from build123d import *

# Parameters (mm, degrees)
F0_W     = 149.987
F0_H     = 69.6976
F1_DEPTH = 25.4
F2_W     = 66.675
F2_H     = 25.2984
F3_DEPTH = 12.7
F5_DEPTH = 12.7
F6_W     = 37.735215
F6_H     = 10.168377
F7_DEPTH = 12.7
F9_DEPTH = 1.3716


with BuildPart() as f1:
    # F0 (on Front) → F1 (new body)
    with BuildSketch(Plane.XZ):
        Rectangle(F0_W, F0_H)
    extrude(amount=F1_DEPTH)

    # F2 (on face) → F3 (cut)
    with BuildSketch(Plane.XZ.offset(25.4)):
        with Locations((0, 22.1996)):
            Rectangle(F2_W, F2_H)
    extrude(amount=-F3_DEPTH, mode=Mode.SUBTRACT)

    # F4 (on face) → F5 (cut)
    with BuildSketch(Plane.XZ.offset(25.4)):
        Polygon((33.3375, 9.5504), (-33.3375, 9.5504), (-74.9935, 15.9512), (-74.9935, -24.998723), (74.9935, -24.998723), (74.9935, 15.9512), align=None)
    extrude(amount=-F5_DEPTH, mode=Mode.SUBTRACT)

    # F6 (on face) → F7 (join)
    with BuildSketch(Plane.XZ.offset(12.7)):
        with Locations((-14.469893, 14.634588)):
            Rectangle(F6_W, F6_H)
    extrude(amount=F7_DEPTH)

    # F8 (on face) → F9 (join)
    with BuildSketch(Plane(origin=(0, 0, 0), x_dir=(-1, 0, 0), z_dir=(0, 1, 0))):
        Polygon((-5.378736, 13.970545), (-13.324757, 27.590852), (-14.065389, 25.489114), (-10.146485, 18.771706), (-11.020009, 17.885251), (-14.361666, 23.663847), (-14.942966, 21.517376), (-11.619632, 15.689826), (-12.511065, 14.787045), (-15.413008, 19.761277), (-16.012603, 17.598834), (-13.045956, 12.513692), (-13.982809, 11.584633), (-16.470851, 15.849397), (-17.257973, 13.296365), (-14.628438, 8.777128), (-15.523009, 7.89), (-17.603708, 11.507705), (-19.224059, 5.78715), (-2.314166, -5.613022), (-2.314166, -7.630318), (-7.419162, -13.35848), (-6.456276, -14.415695), (-3.713523, -11.190438), (-3.327152, -11.61466), (-5.894728, -14.962248), (-4.883376, -15.92657), (-2.861757, -13.310585), (-2.387249, -13.763027), (-4.326059, -16.532207), (-3.442212, -17.475365), (-1.889574, -15.639646), (-1.311372, -16.128685), (-2.922849, -18.03397), (-1.92949, -18.981067), (-1.01934, -17.795069), (-0.374972, -18.382913), (-1.436909, -19.49672), (0.299996, -21.152735), (1.878888, -19.49672), (0.919775, -18.382913), (1.456053, -17.795069), (2.404852, -18.981067), (3.415506, -18.03397), (1.820631, -16.128685), (2.404852, -15.639646), (3.941494, -17.475365), (4.840794, -16.532207), (2.89907, -13.763027), (3.395835, -13.310585), (5.390918, -15.92657), (6.449709, -14.962248), (3.797929, -11.61466), (4.333463, -11.190438), (6.88834, -14.415695), (8.049124, -13.35848), (2.832049, -7.630318), (2.832049, -5.613022), (19.73976, 5.78715), (18.108712, 11.507705), (15.947106, 7.89), (15.048685, 8.777128), (17.748964, 13.296365), (16.968758, 15.849397), (14.510422, 11.584633), (13.569537, 12.513692), (16.607948, 17.598834), (15.947106, 19.761277), (12.974964, 14.787045), (12.060693, 15.689826), (15.542698, 21.517376), (14.857555, 23.663847), (11.526601, 17.885251), (10.627024, 18.771706), (14.432989, 25.489114), (13.762125, 27.590852), (5.914255, 13.976232), (9.222287, 8.290899), (5.935366, 5.0631), (2.720125, 5.0631), (4.767341, 7.097367), (2.442414, 11.553886), (-3.681165, 9.865881), (-0.970141, 7.097367), (-3.078866, 5.03243), (-5.430478, 5.03243), (-8.664062, 8.293143), align=None)
        Polygon((-0.485612, 0.682145), (0, 2.126915), (0.485041, 0.682145), (2.099235, 0.682145), (0.796223, -0.344701), (1.207654, -1.78771), (0, -0.84399), (-1.242889, -1.792924), (-0.851036, -0.344701), (-2.131865, 0.682145), align=None, mode=Mode.SUBTRACT)
    extrude(amount=F9_DEPTH)


solid = f1.part
Geometry check sheet. Reference: the model listing, model coordinates, mm. A direction names the side the tool comes from. Coordinates: 2 decimals unless noted, no trailing zeros. Order: outer loops, then holes, each group sorted by start corner. A loop starts at its lowest first (then second) coordinate and runs counter-clockwise, first axis right, second up. Notation, with made-up numbers: (-6.5, -3.5) - (44.5, -3.5) arc R24 ccw to (44.5, 35.5) - close; hole circle Ø1 at (68.5, 17). An arc over 180 degrees is marked (long way). Answer in a Markdown table with one row per item. Add a question column.
1) Cross-section at D-D, the plane x = -60.5. Record the cut outline in (y, z), then the cut area to 3 significant figures.
2) Cross-section at B-B, the plane x = -27.5. Record the cut outline in (y, z), then the cut area to 3 significant figures.
3) Gauge pin test, flat ends, axial feed: P1, Ø4, axis at x = -23, y = -16.5, coming from the +Z side; P2, Ø1.5, axis at x = 1, y = 1, coming from the -Z side; P3, Ø8, axis at x = 33, z = -7, coming from the -Y side. Record the tip position at first contact, or that the pin passes through.
4) Material ranges on line 1 along X through (y, z) = (-21, 19.5); line 2 along Z through (x, y) = (-17.5, -22.5); line 3 along Z through (x, y) = (64.5, -18.25), recorded low to high. Write a range as [from, to].
5) Release check for a two-part mould opening along X. For faces 5 (the flat face through (-11.17, 0.68, 0.01)), 6 (the flat face through (7.025, 0.676, 6.64)), 7 (the flat face through (54.457, -19.139, 12.796)) record: +X half, -X half, draft (parallel to the pull), parting line (faces both ways), or undercut.
6) Set-up check for faces 1 (the flat face through (-13.8, 0.7, 18.6)), 2 (the flat face through (-15, -19, 19.719)), 3 (the flat face through (-53.874, -19.139, 12.706)), 4 (the flat face through (9.3, 0.68, 20.69)): record each of +Z, -Z, +X, -X, +Y, -Y from which the full face is reachable in a straight line by a thin tool's end or side.
7) Cross-section at A-A, the plane y = -15.75. Record the cut outline in (x, z).
8) Cross-section at C-C, the plane z = -26.5. Record the cut outline in (x, y).
Check result:
| question | item | result |
|---|---|---|
| 1 | outline | (-25.4, -34.85) - (0, -34.85) - (0, 34.85) - (-25.4, 34.85) - (-25.4, 13.72) - (-12.7, 13.72) - (-12.7, -25) - (-25.4, -25) - close |
| 1 | area | 1,280 mm² |
| 2 | outline | (-25.4, -34.85) - (0, -34.85) - (0, 34.85) - (-12.7, 34.85) - (-12.7, 19.72) - (-25.4, 19.72) - (-25.4, 9.55) - (-12.7, 9.55) - (-12.7, -25) - (-25.4, -25) - close |
| 2 | area | 1,140 mm² |
| 3 | P1 | stops at z = 19.72 |
| 3 | P2 | stops at z = -20.63 |
| 3 | P3 | stops at y = -12.7 |
| 4 | line 1 | x = [-74.99, 4.4], [33.34, 74.99] |
| 4 | line 2 | z = [-34.85, -25], [9.55, 19.72] |
| 4 | line 3 | z = [-34.85, -25], [14.34, 34.85] |
| 5 | face 5 | -X half |
| 5 | face 6 | undercut |
| 5 | face 7 | +X half |
| 6 | face 1 | +Y |
| 6 | face 2 | +Z, -Y |
| 6 | face 3 | -X, -Y |
| 6 | face 4 | +Z, +Y |
| 7 | outline | (-74.99, -34.85) - (74.99, -34.85) - (74.99, -25) - (-74.99, -25) - close; (-74.99, 15.95) - (-33.34, 9.55) - (4.4, 9.55) - (4.4, 19.72) - (-33.34, 19.72) - (-33.34, 34.85) - (-74.99, 34.85) - close; (33.34, 9.55) - (74.99, 15.95) - (74.99, 34.85) - (33.34, 34.85) - close |
| 8 | outline | (-74.99, -25.4) - (74.99, -25.4) - (74.99, 0) - (-74.99, 0) - close |
